For this review, take the finished solid that the model builds, in its own axes (mm). A direction names the side the tool comes from. Coordinates: 2 decimals unless noted, no trailing zeros. Loops run counter-clockwise (first coordinate to the right, second up) from the corner with the lowest first, then second, coordinate; pieces in that order, holes last. Notation, with made-up numbers: (73, 82) - (101, 82) arc R21 cw to (101, 97) - close; hole circle Ø11 at (-26, -7). An arc over 180 degrees is marked (long way). Answer as a JSON object with one key per item and string values. Group by question number.
Item 1: Tool access review of faces 1 (the flat face through (-2, 1, -2)), 2 (the cylindrical face through (-0.1, 0.5, -3)): name each direction out of +Z, -Z, +X, -X, +Y, -Y from which nothing blocks a thin tool from reaching the whole face with its end or side.
Item 2: Clearance check with flat-ended pins moving along their axes: pin 1 (3 mm diameter, centred on x = 0, y = 4.5, fed in from -Z); pin 2 (0.6 mm diameter, centred on y = -3.5, z = 1.5, fed in from -X); pin 3 (0.6 mm diameter, centred on x = 0, y = -2, fed in from -Z). State where each tip first meets the part, or that it passes through.
Item 3: To check wall thickness, follow line 1 (Z direction, x = 0.05, y = 2.25); line 2 (X direction, y = -3, z = -1.4); line 3 (Y direction, x = 2.65, z = 0.7). State the ranges of each line that lie inside material, in increasing order.
Item 4: We need section A-A (y = -2). Give the boundary of the cut face in (x, z).
Item 5: We need section C-C (x = 1.1). Give the boundary of the cut face in (y, z) (3 decimals), then the cut area to 3 significant figures.
Item 6: We need section B-B (z = 0). Give the boundary of the cut face in (x, y).
Item 7: We need section D-D (y = 2.25). Give the boundary of the cut face in (x, z), then the cut area to 3 significant figures.
Autodesk Inventor part; units mm, degrees
ref_plane "YZ Plane" through (0, 0, 0) normal (1, 0, 0) x (0, 1, 0)
ref_plane "XZ Plane" through (0, 0, 0) normal (0, 1, 0) x (-1, 0, 0)
ref_plane "XY Plane" through (0, 0, 0) normal (0, 0, 1) x (1, 0, 0)
sketch "Sketch1" plane through (0, 0, 0) normal (0, 1, 0) x (-1, 0, 0)
  arc A0 (-1.6583, 2.5) -> (1.6583, 2.5) centre (0, 0) ccw
  circle A1 centre (0, 0) radius 2.5
  line L0 (0.25, 1.77) -> (-0.25, 1.77)
  line L1 (-0.25, 1.77) -> (-0.25, 1.27)
  line L2 (-0.25, 1.27) -> (0.25, 1.27)
  line L3 (0.25, 1.27) -> (0.25, 1.77)
  line L4 (0, 1.87) -> (0, -2) construction
  line L5 (1.5109, 0) -> (-1.3865, 0) construction
  line L6 (0.25, -1.27) -> (-0.25, -1.27)
  line L7 (-0.25, -1.27) -> (-0.25, -1.77)
  line L8 (-0.25, -1.77) -> (0.25, -1.77)
  line L9 (0.25, -1.77) -> (0.25, -1.27)
  line L10 (-1.6583, 2.5) -> (1.6583, 2.5)
  dimension "d0" = 6
  dimension "d1" = 5
  dimension "d2" = 0.5
  dimension "d4" = 0.5
  dimension "d5" = 2.54
extrude "Extrusion1" add sketch "Sketch1" along normal blind 8.6 contours A1 | L3 L2 L1 L0 | L9 L8 L7 L6
extrude "Extrusion3" add sketch "Sketch1" along normal blind 1 contours L10 A0
fillet "Fillet1" radius 2.5 1 edges at (2.5, 8.6, 0)
extrude "Extrusion4" add sketch "Sketch1" against normal blind 5 contours L3 L2 L1 L0 | L9 L8 L7 L6
properties part number "LED"
Check sheet entries:
{
 "1": {"face 1": "+Y", "face 2": "+Y, -Y"},
 "2": {"pin 1": "stops at z = -2.5", "pin 2": "stops at x = -0.25", "pin 3": "stops at z = -1.77"},
 "3": {"line 1": "z = -2.5 to 2.5", "line 2": "x = -0.25 to 0.25", "line 3": "y = 0 to 1"},
 "4": {"outline": "(-0.25, -1.77) - (0.25, -1.77) - (0.25, -1.27) - (-0.25, -1.27) - close; (-0.25, 1.27) - (0.25, 1.27) - (0.25, 1.77) - (-0.25, 1.77) - close"},
 "5": {"outline": "(0, -2.791) - (1, -2.791) - (1, -2.245) - (6.1, -2.245) arc R2.245 ccw to (6.1, 2.245) - (1, 2.245) - (1, 2.5) - (0, 2.5) - close", "area": "36.1 mm2"},
 "6": {"outline": "(-3, 0) - (3, 0) - (3, 1) - (2.5, 1) - (2.5, 6.1) arc R2.5 ccw to (-2.5, 6.1) - (-2.5, 1) - (-3, 1) - close"},
 "7": {"outline": "circle Ø5 at (0, 0)", "area": "19.6 mm2"}
}
